The listing builds one solid part. Answer for the finished solid, in the listing's coordinates (mm). A direction names the side the tool comes from. Coordinates: 2 decimals unless noted, no trailing zeros. Loops run counter-clockwise (first coordinate to the right, second up) from the corner with the lowest first, then second, coordinate; pieces in that order, holes last. Notation, with made-up numbers: (50, -27) -> (104, -27) arc R30 cw to (104, 9) -> close; hole circle Ø6 at (-23.5, 52.25). An arc over 180 degrees is marked (long way). Answer in a Markdown table with one row per item.
```python
from build123d import *

# Parameters (mm, degrees)
EXTRUDE_1_DEPTH     = 10
SKETCH_4_W          = 10
SKETCH_4_H          = 4
EXTRUDE_2_DEPTH     = 10
CUT_EXTRUDE_1_REACH = 164.425
SKETCH_2_R          = 1.45
FILLET_1_R          = 2
EXTRUDE_3_DEPTH     = 10
FILLET_5_R          = 1.5
EXTRUDE_4_DEPTH     = 10
CUT_EXTRUDE_3_REACH = 174.593
FILLET_3_R          = 3
CHAMFER_1_SIZE      = 7
FILLET_7_R          = 5


with BuildPart() as part:
    # 草图1 → 拉伸-薄壁1 (new body)
    with BuildSketch(Plane(origin=(0, 0, 0), x_dir=(0, 0, -1), z_dir=(1, 0, 0))):
        Polygon((98, -126.439708953), (25, 0), (-25, 0), (-25, 4), (27.309401077, 4), (101.464101615, -124.439708953), align=None)
    extrude(amount=EXTRUDE_1_DEPTH)

    # 草图4 → 凸台-拉伸2 (add)
    with BuildSketch(Plane(origin=(10, 0, 0), x_dir=(0, 0, -1), z_dir=(1, 0, 0))):
        Polygon((27.309401077, 4), (25, 8), (15, 8), (15, 4), align=None)
        with Locations((-20, 6)):
            Rectangle(SKETCH_4_W, SKETCH_4_H)
    extrude(amount=-EXTRUDE_2_DEPTH)

    # 草图2 → 切除-拉伸1 (cut, up to next)
    with BuildSketch(Plane.XZ, mode=Mode.PRIVATE) as cut_extrude_1_sk1:
        with Locations(Location((5, 20, 0), (0, 0, 270))):
            Circle(SKETCH_2_R)
    cut_extrude_1_tool1 = extrude(cut_extrude_1_sk1.sketch, amount=-CUT_EXTRUDE_1_REACH, mode=Mode.PRIVATE) & part.part
    # 草图2 → 切除-拉伸1 (cut, up to next)
    with BuildSketch(Plane.XZ, mode=Mode.PRIVATE) as cut_extrude_1_sk2:
        with Locations(Location((5, -20, 0), (0, 0, 270))):
            Circle(SKETCH_2_R)
    cut_extrude_1_tool2 = extrude(cut_extrude_1_sk2.sketch, amount=-CUT_EXTRUDE_1_REACH, mode=Mode.PRIVATE) & part.part
    add(cut_extrude_1_tool1.solids().sort_by_distance((5, 0, 20))[0], mode=Mode.SUBTRACT)
    add(cut_extrude_1_tool2.solids().sort_by_distance((5, 0, -20))[0], mode=Mode.SUBTRACT)

    # 圆角1
    fillet_1_edges = [part.edges().sort_by_distance(p)[0] for p in [
        (5, 8, 25),
        (5, 4, 15),
        (5, 8, 15),
        (5, 4, -15),
        (5, 8, -15),
        (5, 0, 25),
    ]]
    fillet(fillet_1_edges, radius=FILLET_1_R - 0.0001)  # a hair under: the kernel refuses the full size

    # 草图6 → 凸台-拉伸3 (add)
    with BuildSketch(Plane(origin=(10, 0, 0), x_dir=(0, 0, -1), z_dir=(1, 0, 0))):
        Polygon((25, 8), (40.588457268, 17), (46.088457268, 7.473720558), (43.490381057, 5.973720558), (39.490381057, 12.901923789), (26.5, 5.401923789), align=None)
        Polygon((99.964101615, -121.841632741), (101.464101615, -124.439708953), (117.052558883, -115.439708953), (111.552558883, -105.913429511), (108.954482672, -107.413429511), (112.954482672, -114.341632741), align=None)
    extrude(amount=-EXTRUDE_3_DEPTH)

    # 圆角5
    fillet_5_edges = [part.edges().sort_by_distance(p)[0] for p in [
        (5, -107.413429511, -108.954482672),
        (5, -105.913429511, -111.552558883),
        (5, 5.973720558, -43.490381057),
        (5, 7.473720558, -46.088457268),
    ]]
    fillet(fillet_5_edges, radius=FILLET_5_R - 0.0001)  # a hair under: the kernel refuses the full size

    # 草图7 → 凸台-拉伸4 (add)
    with BuildSketch(Plane(origin=(10, 0, 0), x_dir=(0, 0, -1), z_dir=(1, 0, 0))):
        Polygon((26.5, 5.401923789), (99.964101615, -121.841632741), (102.562177826, -120.341632741), (29.098076211, 6.901923789), align=None)
    extrude(amount=-EXTRUDE_4_DEPTH)

    # 草图8 → 切除-拉伸3 (cut, up to next)
    with BuildSketch(Plane(origin=(10, 0, 0), x_dir=(0, 0, -1), z_dir=(1, 0, 0)), mode=Mode.PRIVATE) as cut_extrude_3_sk1:
        Polygon((25, 0), (98, -126.439708953), (100.598076211, -124.939708953), (28.464101615, 0), align=None)
    cut_extrude_3_tool1 = extrude(cut_extrude_3_sk1.sketch, amount=-CUT_EXTRUDE_3_REACH, mode=Mode.PRIVATE) & part.part
    add(cut_extrude_3_tool1.solids().sort_by_distance((10, -62.8456, -63.01253))[0], mode=Mode.SUBTRACT)

    # 圆角3
    fillet_3_edges = [part.edges().sort_by_distance(p)[0] for p in [
        (5, -115.439708953, -117.052558883),
        (5, -124.939708953, -100.598076211),
        (5, 17, -40.588457268),
    ]]
    fillet(fillet_3_edges, radius=FILLET_3_R)

    # 倒角1
    chamfer_1_edges = [part.edges().sort_by_distance(p)[0] for p in [
        (5, 0, -28.464101615),
    ]]
    chamfer(chamfer_1_edges, length=CHAMFER_1_SIZE)

    # 圆角7
    fillet_7_edges = [part.edges().sort_by_distance(p)[0] for p in [
        (5, -6.062177826, -31.964101615),
    ]]
    fillet(fillet_7_edges, radius=FILLET_7_R)


solid = part.part
```
Item 1: Find the intervals of material crossed by probe 1 along X at (y, z) = (3, 20); probe 2 along Y at (x, z) = (9.5, -44); probe 3 along Y at (x, z) = (3.25, -33.5), in increasing order.
Findings below:
| item | result |
|---|---|
| probe 1 | x = 0 to 3.55, 6.45 to 10 |
| probe 2 | y = -26.91 to -18.91, 6.52 to 11.09 |
| probe 3 | y = -8.72 to -0.72, 9.44 to 12.91 |
Item 2: Determine the mould class of faces 5 (the face through (5.07, -117.3, -107.83)), 6 (the face through (5.07, -2.734, -26.199)), 7 (the face through (5.07, -120.235, -108.747)) for opening direction Z: +Z half, -Z half, draft (parallel to the pull), parting line (faces both ways), or undercut.
Findings below:
| item | result |
|---|---|
| face 5 | undercut |
| face 6 | +Z half |
| face 7 | -Z half |
Item 3: A cutting plane is placed at A-A, the plane y = -16.5. Determine the outline of the cut face in (x, z), plus the area to 3 significant figures.
Findings below:
| item | result |
|---|---|
| outline | (0, -42.61) -> (10, -42.61) -> (10, -37.99) -> (0, -37.99) -> close |
| area | 46.2 mm2 |
Item 4: Flat-ended cylindrical pins translate along their axes: pin 1 Ø5 at (x, y) = (8.5, -105.5) entering from -Z; pin 2 Ø6 at (x, y) = (1.5, -69) entering from +Z; pin 3 Ø5 at (x, z) = (3.5, -7.5) entering from -Y. Find the tip coordinate at first contact, or state that the pin passes through.
Findings below:
| item | result |
|---|---|
| pin 1 | stops at z = -112.76 |
| pin 2 | stops at z = -66.57 |
| pin 3 | stops at y = 0 |
Item 5: A tool of negligible diameter and unlimited length cuts with its end or side. For faces 1 (the face through (5.07, -111.49, -111.31)), 2 (the face through (5, 4, 0)), 3 (the face through (5, 8, -22)), 4 (the face through (5, 0, 0)), from which of +Z, -Z, +X, -X, +Y, -Y can it reach the whole face along a straight path? Write none if from no direction.
Findings below:
| item | result |
|---|---|
| face 1 | +X, -X |
| face 2 | +X, -X, +Y |
| face 3 | +Z, +X, -X, +Y |
| face 4 | +Z, +X, -X, -Y |
